Can you work these out from the drawing? Everything is in mm from the part's minimum corner. A direction names the side the tool comes from. Coordinates: 2 decimals unless noted, no trailing zeros. Order: outer loops, then holes, each group sorted by start corner. A loop starts at its lowest first (then second) coordinate and runs counter-clockwise, first axis right, second up. Notation, with made-up numbers: (59, 14.5) -> (77, 14.5) arc R21 cw to (77, 53.5) -> close; hole circle Ø7 at (47, 26). An arc over 180 degrees is marked (long way). Use a Markdown table: item, result. Add a question column.
1) Will these pins go through, and if not, where does the flat tip stop? pin 1 Ø11 at (x, z) = (30, 30) entering from -Y; pin 2 Ø8 at (x, y) = (11.5, 21) entering from +Z; pin 3 Ø1.5 at (y, z) = (15, 45) entering from -X; pin 4 Ø10 at (x, y) = (47, 14.5) entering from -Z.
2) If we section it at A-A (z = 30): Write out the boundary of the cut face in (x, y).
3) If I drill on L1, parallel to Z at x = 50, y = 35.25; L2, parallel to X at y = 28.5, z = 29.5; L3, parallel to Y at x = 22.5, z = 12.5, over which ranges is the centre line in solid material (lowest first)? Write a range as [from, to].
4) If we section it at C-C (x = 30): Write out the boundary of the cut face in (y, z), plus the area to 3 significant figures.
5) If we section it at B-B (y = 36): Write out the boundary of the cut face in (x, z).
6) If we section it at D-D (z = 47): Write out the boundary of the cut face in (x, y), plus the area to 3 significant figures.
7) Thinking about a two-plate mould opening in Z: for the marked faces 1, 2 and 3, which applies, +Z half, -Z half, draft (parallel to the pull), parting line (faces both ways), or undercut?
8) Which directions (+Z, -Z, +X, -X, +Y, -Y) give clear straight access to the entire face, cutting with the end or side of a thin tool? Please do the marked faces 4 and 5.
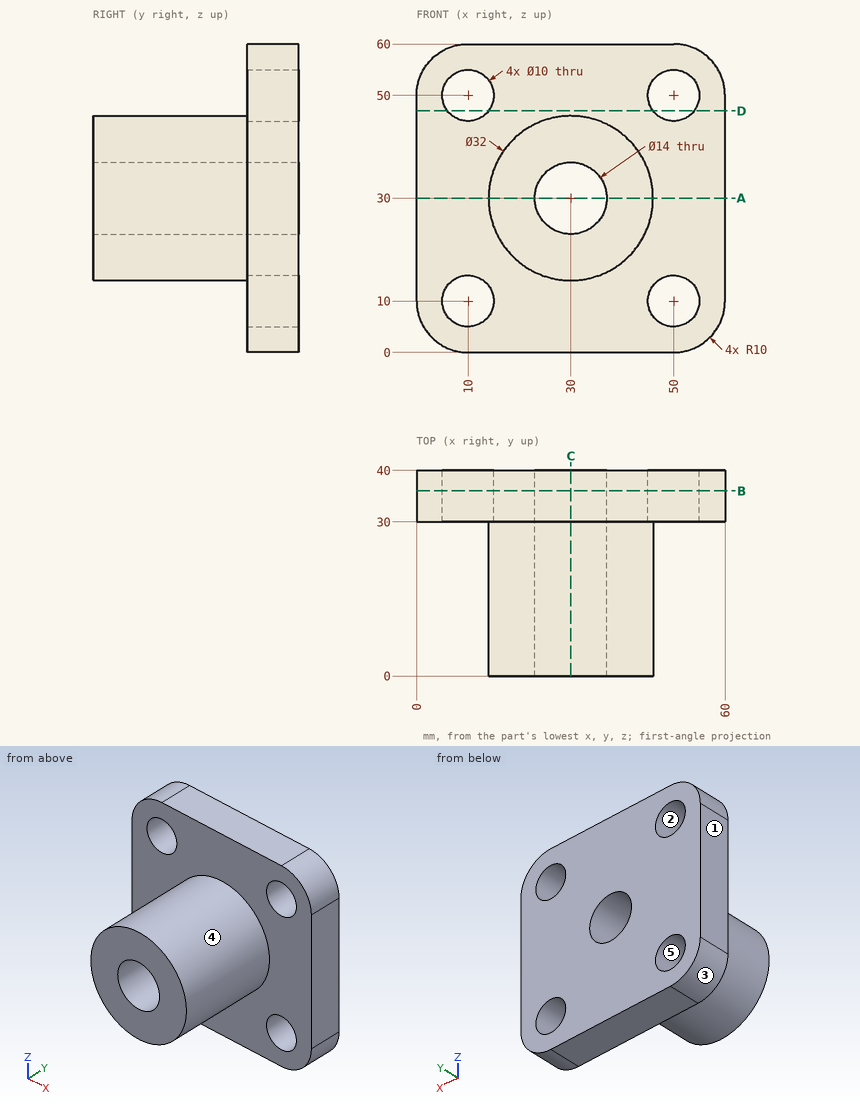
Answer sheet:
| question | item | result |
|---|---|---|
| 1 | pin 1 | through |
| 1 | pin 2 | z = 36.76 |
| 1 | pin 3 | x = 22.72 |
| 1 | pin 4 | z = 19.42 |
| 2 | outline | (0, 30) -> (14, 30) -> (14, 0) -> (23, 0) -> (23, 40) -> (0, 40) -> close; (37, 0) -> (46, 0) -> (46, 30) -> (60, 30) -> (60, 40) -> (37, 40) -> close |
| 3 | L1 | [0, 5], [15, 45], [55, 60] |
| 3 | L2 | [14.01, 23.02], [36.98, 45.99] |
| 3 | L3 | [30, 40] |
| 4 | outline | (0, 14) -> (30, 14) -> (30, 0) -> (40, 0) -> (40, 23) -> (0, 23) -> close; (0, 37) -> (40, 37) -> (40, 60) -> (30, 60) -> (30, 46) -> (0, 46) -> close |
| 4 | area | 1,000 mm2 |
| 5 | outline | (0, 10) arc R10 ccw to (10, 0) -> (50, 0) arc R10 ccw to (60, 10) -> (60, 50) arc R10 ccw to (50, 60) -> (10, 60) arc R10 ccw to (0, 50) -> close; hole circle Ø10 at (10, 10); hole circle Ø10 at (10, 50); hole circle Ø14 at (30, 30); hole circle Ø10 at (50, 10); hole circle Ø10 at (50, 50) |
| 6 | outline | (0, 30) -> (6, 30) -> (6, 40) -> (0, 40) -> close; (14, 30) -> (46, 30) -> (46, 40) -> (14, 40) -> close; (54, 30) -> (60, 30) -> (60, 40) -> (54, 40) -> close |
| 6 | area | 440 mm2 |
| 7 | face 1 | draft |
| 7 | face 2 | undercut |
| 7 | face 3 | -Z half |
| 8 | face 4 | -Y |
| 8 | face 5 | +Y, -Y |
